Design review of the part shown in the three views and the two pictorial views. Dimensions are in mm from the part's minimum x, y and z. A direction names the side the tool comes from. Coordinates: 2 decimals unless noted, no trailing zeros. Write each loop counter-clockwise with the first axis right and the second up, starting at its lowest first coordinate (ties: lowest second). Pieces come first, ordered by that corner, then holes. Notation, with made-up numbers: (-7, 78.5) -> (23, 78.5) arc R17 cw to (23, 95.5) -> close; hole circle Ø5 at (87, 7.25). An arc over 180 degrees is marked (long way). Write each question's results on one line, items separated by ' | '.
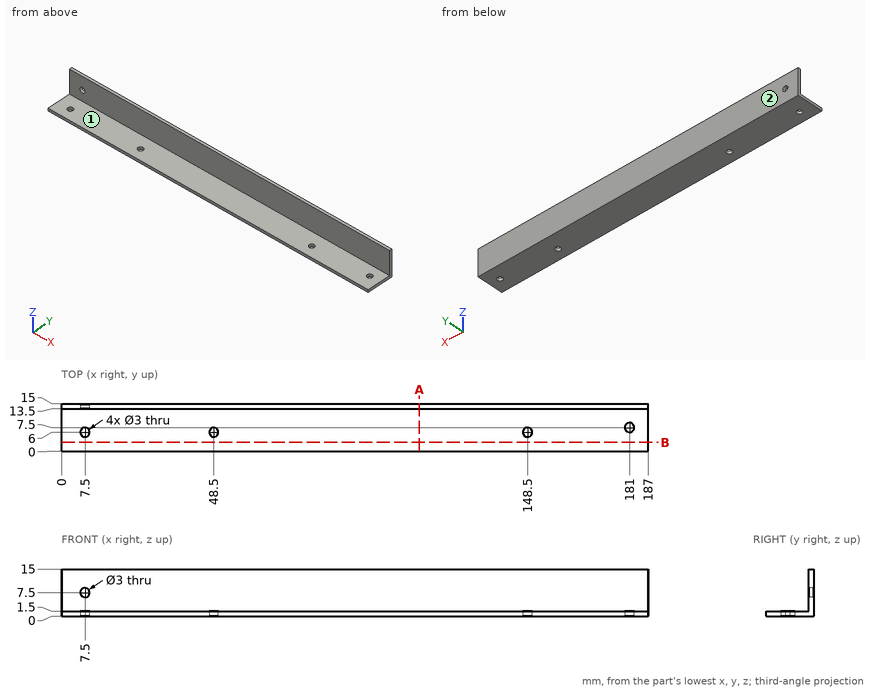
Q1. Clearance check with flat-ended pins moving along their axes: P1, Ø6, axis at x = 157, z = 13.5, coming from the -Y side; P2, Ø5, axis at x = 48.5, y = 6, coming from the +Z side. State where each tip first meets the part, or that it passes through.
Solution:
P1: y = 13.5 | P2: z = 1.5
Q2. Machinability: for the marked faces 1 and 2, which of the approach directions +Z, -Z, +X, -X, +Y, -Y give a long, thin tool a straight path to every point of the face, cutting with its end or side? Answer none if there is none.
Solution:
face 1: +Z, +X, -X, -Y | face 2: +Z, -Z, +X, -X, +Y
Q3. Add section A-A (x = 114). Write out the cut boundary in (y, z), plus the area to 4 significant figures.
Solution:
outline: (0, 0) -> (15, 0) -> (15, 15) -> (13.5, 15) -> (13.5, 1.5) -> (0, 1.5) -> close | area: 42.75 mm²
Q4. For line 1 (Z direction, x = 7.5, y = 14); line 2 (Y direction, x = 148.5, z = 0.9); line 3 (Y direction, x = 28.5, z = 7), list the stretches that pass through material, from the lowest coordinate up. Write a range as from..to.
Solution:
line 1: 0..6, 9..15 | line 2: 0..4.5, 7.5..15 | line 3: 13.5..15
Q5. Add section B-B (y = 2.75). Write out the cut boundary in (x, z).
Solution:
outline: (0, 0) -> (187, 0) -> (187, 1.5) -> (0, 1.5) -> close
